Input: dimensioned drawing with shaded views. Units: mm. Origin: part minimum x, y, z. A direction names the side the tool comes from. Round coordinates to 2 decimals unless told otherwise and drop trailing zeros. Loops run counter-clockwise (first coordinate to the right, second up) from the corner with the lowest first, then second, coordinate; pieces in that order, holes last. Notation, with made-up numbers: (40, 26.5) -> (68, 26.5) arc R17 cw to (68, 36.5) -> close; hole circle Ø9 at (-2, 84.5). An arc over 180 degrees is marked (long way). Answer as a JSON object with one key per item and string values.
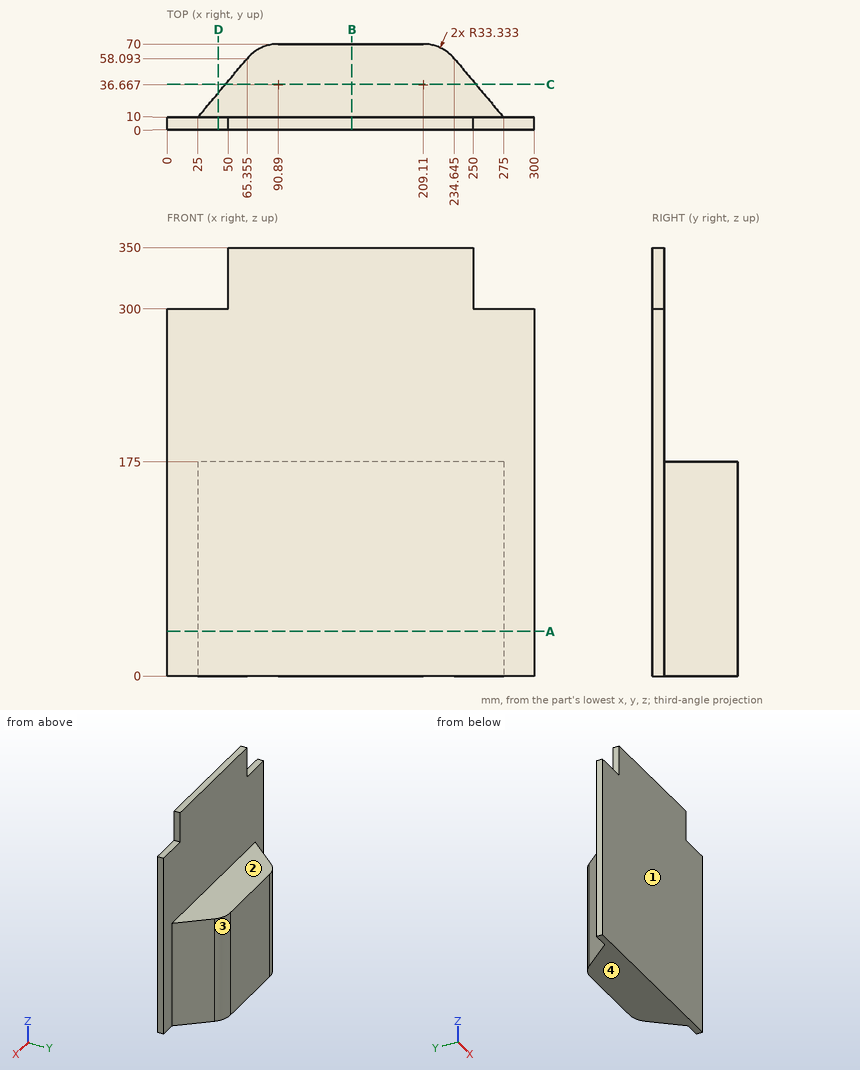
1) Section C-C, the plane y = 37. Output: boundary loops of the cut face in (x, z) (1 decimal).
Output:
{"outline": "(47.7, 0) -> (252.3, 0) -> (252.3, 175) -> (47.7, 175) -> close"}
2) Reachability of the marked faces 1 and 2 from +Z, -Z, +X, -X, +Y, -Y: full face, straight path, thin tool, end or side. Return the list, or none.
Output:
{"face 1": "+Z, -Z, +X, -X, -Y", "face 2": "+Z, +X, -X, +Y"}
3) Section B-B, the plane x = 151. Output: boundary loops of the cut face in (y, z).
Output:
{"outline": "(0, 0) -> (70, 0) -> (70, 175) -> (10, 175) -> (10, 350) -> (0, 350) -> close"}
4) Draft query along X for the marked faces 3 and 4. Return one class per face: +X half, -X half, draft (parallel to the pull), parting line (faces both ways), or undercut.
Output:
{"face 3": "+X half", "face 4": "draft"}
5) Section A-A, the plane z = 36.5. Output: boundary loops of the cut face in (x, y) (1 decimal).
Output:
{"outline": "(0, 0) -> (300, 0) -> (300, 10) -> (275, 10) -> (234.6, 58.1) arc R33.3 ccw to (209.1, 70) -> (90.9, 70) arc R33.3 ccw to (65.4, 58.1) -> (25, 10) -> (0, 10) -> close"}
6) Section D-D, the plane x = 42. Output: boundary loops of the cut face in (y, z).
Output:
{"outline": "(0, 0) -> (30.26, 0) -> (30.26, 175) -> (10, 175) -> (10, 300) -> (0, 300) -> close"}
7) Contact query for flat-ended pins moving along their axis: P1, Ø5, axis at y = 6, z = 316, coming from the -X side; P2, Ø10, axis at x = 139.5, z = 220, coming from the +Y side; P3, Ø11, axis at x = 13.5, y = 4, coming from the +Z side. Output: stop coordinate, or through.
Output:
{"P1": "stops at x = 50", "P2": "stops at y = 10", "P3": "stops at z = 300"}
8) Ray query, probe 1 along Y at (x, z) = (189, 211); probe 2 along Z at (x, y) = (248, 40.5); probe 3 along Z at (x, y) = (276.5, 9). Return the intervals inside material, ascending.
Output:
{"probe 1": "y = 0 to 10", "probe 2": "z = 0 to 175", "probe 3": "z = 0 to 300"}
